Autodesk Inventor part; units mm, degrees
ref_plane "YZ Plane" through (0, 0, 0) normal (1, 0, 0) x (0, 1, 0)
ref_plane "XZ Plane" through (0, 0, 0) normal (0, 1, 0) x (-1, 0, 0)
ref_plane "XY Plane" through (0, 0, 0) normal (0, 0, 1) x (1, 0, 0)
sketch "Szkic1" plane through (0, 0, 0) normal (0, 0, 1) x (1, 0, 0)
  line L0 (-28.5, -28.5) -> (28.5, -28.5)
  line L1 (28.5, -28.5) -> (28.5, 28.5)
  line L2 (28.5, 28.5) -> (-28.5, 28.5)
  line L3 (-28.5, 28.5) -> (-28.5, -28.5)
  line L4 (-28.5, -28.5) -> (28.5, 28.5) construction
  line L5 (28.5, -28.5) -> (-28.5, 28.5) construction
  line L6 (-28.5, 20.9975) -> (-20.9975, 28.5)
  line L7 (20.9975, 28.5) -> (28.5, 20.9975)
  line L8 (28.5, -20.9975) -> (20.9975, -28.5)
  line L9 (-20.9975, -28.5) -> (-28.5, -20.9975)
  line L10 (0, 32.5269) -> (0, -32.5269) construction
  point P0 (0, 0)
  dimension "d0" = 57
  dimension "d3" = 70
  dimension "d4" = 70
extrude "Wyciągnięcie proste1" add sketch "Szkic1" along normal blind 45 contours L9 L3 L6 L2 L7 L1 L8 L0
sketch "Szkic2" plane through (0, 0, 45) normal (0, 0, 1) x (1, 0, 0)
  line L0 (20.9975, -28.5) -> (28.5, -20.9975)
  line L1 (28.5, -20.9975) -> (28.5, 20.9975)
  line L2 (28.5, 20.9975) -> (20.9975, 28.5)
  line L3 (20.9975, 28.5) -> (-20.9975, 28.5)
  line L4 (-20.9975, 28.5) -> (-28.5, 20.9975)
  line L5 (-28.5, 20.9975) -> (-28.5, -20.9975)
  line L6 (-28.5, -20.9975) -> (-20.9975, -28.5)
  line L7 (-20.9975, -28.5) -> (20.9975, -28.5)
  line L8 (20.9975, 28.5) -> (-20.9975, 28.5)
  line L9 (13.9264, 28.5) -> (28.5, 13.9264)
  line L10 (28.5, -20.9975) -> (28.5, 20.9975)
  line L11 (13.9264, -28.5) -> (28.5, -13.9264)
  line L12 (-20.9975, -28.5) -> (20.9975, -28.5)
  line L13 (-13.9264, -28.5) -> (-28.5, -13.9264)
  line L14 (-28.5, 20.9975) -> (-28.5, -20.9975)
  line L15 (-28.5, 13.9264) -> (-13.9264, 28.5)
  line L16 (-28.5, -20.9975) -> (-20.9975, -28.5) construction
  line L17 (-24.7487, -24.7487) -> (24.7487, 24.7487) construction
  line L18 (20.9975, -28.5) -> (28.5, -20.9975) construction
  line L19 (24.7487, -24.7487) -> (-24.7487, 24.7487) construction
  line L20 (-20.9975, 28.5) -> (-28.5, 20.9975) construction
  line L21 (-28.5, -20.9975) -> (-20.9975, -28.5) construction
  line L22 (28.5, 20.9975) -> (20.9975, 28.5) construction
  point P0 (0, 0)
  dimension "d7" = 60
  dimension "d8" = 60
extrude "Wyciągnięcie proste2" add sketch "Szkic2" along normal blind 6 contours L7 L13 L5 L15 L3 L9 L1 L11
sketch "Szkic3" plane through (0, 0, 51) normal (0, 0, 1) x (1, 0, 0)
  line L0 (20.9975, -28.5) -> (28.5, -20.9975)
  line L1 (-20.9975, -28.5) -> (20.9975, -28.5)
  line L2 (-28.5, -20.9975) -> (-20.9975, -28.5)
  line L3 (-28.5, 20.9975) -> (-28.5, -20.9975)
  line L4 (-20.9975, 28.5) -> (-28.5, 20.9975)
  line L5 (20.9975, 28.5) -> (-20.9975, 28.5)
  line L6 (28.5, 20.9975) -> (20.9975, 28.5)
  line L7 (28.5, -20.9975) -> (28.5, 20.9975)
  line L8 (-28.5, -28.5) -> (28.5, -28.5)
  line L9 (28.5, -28.5) -> (28.5, 28.5)
  line L10 (28.5, 28.5) -> (-28.5, 28.5)
  line L11 (-28.5, 28.5) -> (-28.5, -28.5)
  point P0 (0, 0)
  point P1 (0, 28.5)
  point P2 (28.5, 0)
  point P3 (0, -28.5)
extrude "Wyciągnięcie proste3" add sketch "Szkic3" along normal blind 4.8
sketch "Szkic4" plane through (0, 0, 55.8) normal (0, 0, 1) x (1, 0, 0)
  circle A0 centre (0, 0) radius 19.05
  dimension "d13" = 38.1
extrude "Wyciągnięcie proste4" add sketch "Szkic4" along normal blind 2.5
sketch "Szkic5" plane through (0, 0, 55.8) normal (0, 0, 1) x (1, 0, 0)
  line L0 (-23.57, -23.57) -> (23.57, -23.57) construction
  line L1 (23.57, -23.57) -> (23.57, 23.57) construction
  line L2 (23.57, 23.57) -> (-23.57, 23.57) construction
  line L3 (-23.57, 23.57) -> (-23.57, -23.57) construction
  line L4 (-23.57, -23.57) -> (23.57, 23.57) construction
  line L5 (23.57, -23.57) -> (-23.57, 23.57) construction
  point P0 (0, 0)
  dimension "d16" = 47.14
hole "Otwór1" at (-23.57, 23.57, 55.8) at (23.57, 23.57, 55.8) at (23.57, -23.57, 55.8) at (-23.57, -23.57, 55.8) direction (0, 0, -1) diameter 5 depth 5
sketch "Szkic6" plane through (0, 0, 58.3) normal (0, 0, 1) x (1, 0, 0)
  circle A0 centre (0, 0) radius 5
  dimension "d24" = 10
extrude "Wyciągnięcie proste5" cut sketch "Szkic6" against normal up to surface (2.5 mm away)
sketch "Szkic7" plane through (0, 0, 55.8) normal (0, 0, 1) x (1, 0, 0)
  circle A0 centre (0, 0) radius 5
  circle A1 centre (0, 0) radius 3.175
  dimension "d27" = 6.35
extrude "Wyciągnięcie proste6" add sketch "Szkic7" along normal blind 21 contours A1
sketch "Szkic8" plane through (0, 0, 76.8) normal (0, 0, 1) x (1, 0, 0)
  circle A0 centre (0, 0) radius 3.175
  line L0 (-2.4659, 2) -> (2.4659, 2)
  dimension "d30" = 2
extrude "Wyciągnięcie proste7" cut sketch "Szkic8" against normal blind 19 contours L0 A0 picked at (-0.6547, 2.1648)
sketch "Szkic9" plane through (0, 0, 76.8) normal (0, 0, 1) x (1, 0, 0)
  point P0 (0, 0)
  point P1 (0, 0)
hole "Otwór2" at (0, 0, 76.8) direction (0, 0, -1) diameter 2.5 depth 2 tip angle 118
fillet "Zaokrąglenie1" radius 2 4 edges at (28.5, -28.5, 53.4) (28.5, 28.5, 53.4) (-28.5, 28.5, 53.4) (-28.5, -28.5, 53.4)
properties part number "stepper"
Design review of the part built by this model. Coordinates are the model's own, in mm. A direction names the side the tool comes from. Round coordinates to 2 decimals unless told otherwise and drop trailing zeros. Write each loop counter-clockwise with the first axis right and the second up, starting at its lowest first coordinate (ties: lowest second). Pieces come first, ordered by that corner, then holes. Notation, with made-up numbers: (-4, 17.25) -> (33, 17.25) arc R18 ccw to (33, 38.25) -> close; hole circle Ø8 at (30.25, 47). An arc over 180 degrees is marked (long way). One line per item, written item: value. Start each with the question number.
Q1. Add section B-B (z = 54.5). Give the boundary of the cut face in (x, y).
Q2. To check wall thickness, follow probe 1 along Y at (x, z) = (-23.57, 53.7); probe 2 along Y at (x, z) = (0, 57.15) (3 decimals). State the ranges of each line that lie inside material, in increasing order.
Q3. The part is to be moulded in two halves that separate along X. For faces 4 (the face through (26.01, 24.11, 53.37)), 5 (the face through (4, -4, 58.3)), 6 (the face through (-24.8, 24.7, 22.2)), say which applies: pulls with the +X half, pulls with the -X half, needs draft (parallel to the pull), parting line crosses it, or undercut.
Q4. Tool access review of faces 1 (the face through (-21.111, -21.315, 47.958)), 2 (the face through (25, 21, 51)), 3 (the face through (-15.12, 11.59, 57.03)): name each direction out of +Z, -Z, +X, -X, +Y, -Y from which nothing blocks a thin tool from reaching the whole face with its end or side.
Q5. Insertion check: P1, Ø6, axis at x = 23.57, y = -23.57, coming from the +Z side; P2, Ø6, axis at x = 3.5, y = -6.5, coming from the +Z side; P3, Ø4, axis at x = 23.57, y = 23.57, coming from the +Z side. Each pin has a flat end and moves straight along its axis. Give the tip position at first contact, or say it passes through.
Q6. Add section A-A (x = -23.57). Give the boundary of the cut face in (y, z), then the cut area to 3 significant figures.
Q7. Add section D-D (z = 26). Give the boundary of the cut face in (x, y).
Response:
1. outline: (-28.5, -26.5) arc R2 ccw to (-26.5, -28.5) -> (26.5, -28.5) arc R2 ccw to (28.5, -26.5) -> (28.5, 26.5) arc R2 ccw to (26.5, 28.5) -> (-26.5, 28.5) arc R2 ccw to (-28.5, 26.5) -> close; hole circle Ø5 at (-23.57, -23.57); hole circle Ø5 at (-23.57, 23.57); hole circle Ø5 at (23.57, -23.57); hole circle Ø5 at (23.57, 23.57)
2. probe 1: y = -28.5 to -26.07, -21.07 to 21.07, 26.07 to 28.5
2. probe 2: y = -19.05 to -5, -3.175 to 3.175, 5 to 19.05
3. face 4: undercut
3. face 5: needs draft
3. face 6: pulls with the -X half
4. face 1: -X, -Y
4. face 2: +X, +Y
4. face 3: +Z
5. P1: stops at z = 55.8
5. P2: stops at z = 58.3
5. P3: stops at z = 45
6. outline: (-28.5, 51) -> (-26.07, 51) -> (-26.07, 55.8) -> (-28.5, 55.8) -> close; (-25.93, 0) -> (25.93, 0) -> (25.93, 45) -> (18.86, 45) -> (18.86, 51) -> (21.07, 51) -> (21.07, 55.8) -> (-21.07, 55.8) -> (-21.07, 51) -> (-18.86, 51) -> (-18.86, 45) -> (-25.93, 45) -> close; (26.07, 51) -> (28.5, 51) -> (28.5, 55.8) -> (26.07, 55.8) -> close
6. area: 2,790 mm^2
7. outline: (-28.5, -21) -> (-21, -28.5) -> (21, -28.5) -> (28.5, -21) -> (28.5, 21) -> (21, 28.5) -> (-21, 28.5) -> (-28.5, 21) -> close
